Build history of the part. All positions in model axes, mm. Give positions to 0.01 mm unless a question says otherwise; leave off trailing zeros. Write each loop counter-clockwise with the first axis right and the second up, starting at its lowest first coordinate (ties: lowest second). Pieces come first, ordered by that corner, then holes. Notation, with made-up numbers: (89, 70) -> (115, 70) arc R4 cw to (115, 74) -> close; hole circle Ø1 at (83, -15). An arc over 180 degrees is marked (long way). Write item = value, one per line. Start each with the question number.
Q1. Mould opens along X. For faces 1 (the face through (0, 152.4, -2)), 2 (the face through (1.216, 147.571, -1.115)), 3 (the face through (-0.54, 6.44, 2.44)), 4 (the face through (2.243, 152.201, 4.313)) say: pulls with the +X half, pulls with the -X half, needs draft (parallel to the pull), parting line crosses it, or undercut.
Q2. Drop flat-ended pins along their axis: P1, Ø4.5, axis at x = 0, z = 0, coming from the -Y side; P2, Ø4, axis at x = -4, y = 49.5, coming from the +Z side; P3, Ø6, axis at y = 24, z = 4, coming from the -X side. Give the stop position or say it passes through.
Q3. Saw through at A-A, the plane y = 34. List the corners of the cut face in (x, z).
Q4. Wall check: line 1 (X direction, y = 101.5, z = 0.5); line 2 (Z direction, x = -1.75, y = 60); line 3 (Y direction, x = -4.5, z = 3.25). Give the ranges that are in metal, low to high.
from build123d import *

# Parameters (mm, degrees)
SKETCH1_R                 = 6.35
POSTBODY_DEPTH            = 152.4
M4X0_7_TAPPED_HOLE1_D     = 3.3
M4X0_7_TAPPED_HOLE1_DEPTH = 9.525
M4X0_7_TAPPED_HOLE1_TIP   = 0.991420021
M6X1_0_TAPPED_HOLE1_D     = 5
M6X1_0_TAPPED_HOLE1_DEPTH = 12.7
M6X1_0_TAPPED_HOLE1_TIP   = 1.502151548


with BuildPart() as part:
    # Sketch1 → PostBody (new body)
    with BuildSketch(Plane(origin=(0, 0, 0), x_dir=(1, 0, 0), z_dir=(0, 1, 0))):
        with Locations(Location((0, 0, 0), (0, 0, 90))):
            Circle(SKETCH1_R)
    extrude(amount=POSTBODY_DEPTH)

    # TopCut: sweep along a path in Sketch5
    with BuildLine(Plane(origin=(0, 152.4, 0), x_dir=(1, 0, 0), z_dir=(0, 1, 0))) as topcut_path:
        CenterArc((0, 0), 4.748740119, 0, 360)
    # Sketch4 → TopCut (sweep, cut)
    with BuildSketch(Plane.XY):
        Polygon((6.35, 152.4), (6.35, 149.225), (4.7625, 152.4), align=None)
    sweep(path=topcut_path.line, mode=Mode.SUBTRACT)

    # M4x0.7 Tapped Hole1
    with Locations(Plane(origin=(0, 152.4, 0), x_dir=(1, 0, 0), z_dir=(0, 1, 0))):
        with Locations((0, 0)):
            Hole(M4X0_7_TAPPED_HOLE1_D / 2, depth=M4X0_7_TAPPED_HOLE1_DEPTH)
            with Locations((0, 0, -(M4X0_7_TAPPED_HOLE1_DEPTH + M4X0_7_TAPPED_HOLE1_TIP / 2))):  # 118° drill point
                Cone(0, M4X0_7_TAPPED_HOLE1_D / 2, M4X0_7_TAPPED_HOLE1_TIP, mode=Mode.SUBTRACT)

    # M6x1.0 Tapped Hole1
    with Locations(Plane(origin=(0, 0, 0), x_dir=(-1, 0, 0), z_dir=(0, -1, 0))):
        with Locations((0, 0)):
            Hole(M6X1_0_TAPPED_HOLE1_D / 2, depth=M6X1_0_TAPPED_HOLE1_DEPTH)
            with Locations((0, 0, -(M6X1_0_TAPPED_HOLE1_DEPTH + M6X1_0_TAPPED_HOLE1_TIP / 2))):  # 118° drill point
                Cone(0, M6X1_0_TAPPED_HOLE1_D / 2, M6X1_0_TAPPED_HOLE1_TIP, mode=Mode.SUBTRACT)


solid = part.part
Report:
q1.face_1 = needs draft
q1.face_2 = undercut
q1.face_3 = undercut
q1.face_4 = parting line crosses it
q2.P1 = 12.85
q2.P2 = 6.03
q2.P3 = -6.27
q3.outline = circle Ø12.7 at (0, 0)
q4.line_1 = -6.33 to 6.33
q4.line_2 = -6.1 to 6.1
q4.line_3 = 0 to 150.82
